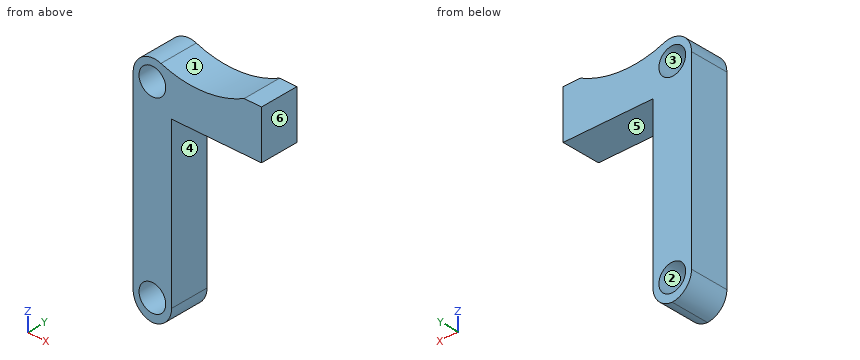
from build123d import *

# Parameters (mm, degrees)
SKETCH1_R           = 3.302
BOSS_EXTRUDE1_DEPTH = 9.525
FILLET1_R           = 5.08
FILLET2_R           = 5.08
FILLET3_DEPTH       = 9.525


with BuildPart() as part:
    # Sketch1 → Boss-Extrude1 (new body)
    with BuildSketch(Plane(origin=(0, 0, 0), x_dir=(1, 0, 0), z_dir=(0, 1, 0))):
        with BuildLine():
            Line((-4.7625, 28.575), (4.7625, 28.575))
            Line((4.7625, 28.575), (4.7625, -17.145))
            Line((4.7625, -17.145), (26.9875, -17.145))
            Line((26.9875, -17.145), (26.9875, -29.1465))
            Line((26.9875, -29.1465), (22.703516651, -29.1465))
            ThreePointArc((22.703516651, -29.1465), (11.1125, -26.347569289), (-0.478516651, -29.1465))
            Line((-0.478516651, -29.1465), (-4.7625, -29.1465))
            Line((-4.7625, -29.1465), (-4.7625, 28.575))
        make_face()
        with Locations(Location((0, -23.241, 0), (0, 0, 90))):
            Circle(SKETCH1_R, mode=Mode.SUBTRACT)
        with Locations(Location((0, 23.241, 0), (0, 0, 90))):
            Circle(SKETCH1_R, mode=Mode.SUBTRACT)
    extrude(amount=BOSS_EXTRUDE1_DEPTH)

    # Fillet1
    # the kernel refuses this fillet: 5.08 mm, written as the material it takes off along each edge
    with BuildSketch(Plane(origin=(-4.7625, -12.7, -28.575), x_dir=(0, 0, 1), z_dir=(0, 1, 0)), Plane(origin=(4.7625, -12.7, -28.575), x_dir=(-1, 0, 0), z_dir=(0, 1, 0))) as fillet1_piece_1:
        with BuildLine():
            CenterArc((FILLET1_R, FILLET1_R), FILLET1_R, 180, 90)
            Line((0, FILLET1_R), (0, 0))
            Line((0, 0), (FILLET1_R, 0))
        make_face()
    extrude(amount=34.925, mode=Mode.SUBTRACT)

    # Fillet2
    # the kernel refuses this fillet: 5.08 mm, written as the material it takes off along each edge
    with BuildSketch(Plane(origin=(-4.7625, -12.543115017, 29.1465), x_dir=(1, 0, 0), z_dir=(0, 1, 0))) as fillet2_piece_1:
        with BuildLine():
            CenterArc((5.08, 5.017246007), FILLET2_R, 180, 80.98481696)
            Line((0, 5.017246007), (-0.1016, 5.017246007))
            Line((-0.1016, 5.017246007), (-0.1016, 0))
            Line((-0.1016, 0), (0, -0.1016))
            ThreePointArc((0, -0.1016), (2.141991675, -0.1016), (4.268063016, -0.10034492))
            Line((4.268063016, -0.10034492), (4.283983349, 0))
        make_face()
    extrude(amount=34.611230034, mode=Mode.SUBTRACT)

    # Fillet3: read off the stored shape, not the designer's step
    # Fillet3 outline → Fillet3 (cut)
    with BuildSketch(Plane(origin=(0, 0, 0), x_dir=(1, 0, 0), z_dir=(0, 1, 0))):
        with BuildLine():
            ThreePointArc((-0.478516651, -29.1465), (0.802955992, -28.533924544), (2.116666667, -27.993938353))
            ThreePointArc((2.116666667, -27.993938353), (-2.569248459, -27.423293904), (-4.7625, -23.243212166))
            Line((-4.7625, -23.243212166), (-4.7625, -24.129253993))
            ThreePointArc((-4.7625, -24.129253993), (-3.545799405, -27.427938232), (-0.478516651, -29.1465))
        make_face()
    extrude(amount=FILLET3_DEPTH, mode=Mode.SUBTRACT)


solid = part.part
Design review of the part built by this model. Coordinates are the model's own, in mm. Face numbers are marked on the shaded views. A direction names the side the tool comes from. Coordinates: 2 decimals unless noted, no trailing zeros. Order: outer loops, then holes, each group sorted by start corner. A loop starts at its lowest first (then second) coordinate and runs counter-clockwise, first axis right, second up.
Item 1: Take a section at C-C, the plane x = 24. Write out the cut boundary in (y, z) (1 decimal).
Item 2: Take a section at D-D, the plane z = 3.5. Write out the cut boundary in (x, y) (1 decimal).
Item 3: For line 1 (Z direction, x = 1, y = 4.75); line 2 (X direction, y = 2, z = -23); line 3 (X direction, y = 4, z = -12.5), list the stretches that pass through material, from the lowest coordinate up.
Item 4: The part is to be moulded in two halves that separate along Z. For the marked faces 1, 2, 3 and 4, say which applies: pulls with the +Z half, pulls with the -Z half, needs draft (parallel to the pull), parting line crosses it, or undercut.
Item 5: Take a section at A-A, the plane y = 3.5. Write out the cut boundary in (x, z) (1 decimal), then the cut area to 3 significant figures.
Item 6: For the marked faces 5 and 6, list the 3-axis set-ups (+Z, -Z, +X, -X, +Y, -Y) from which the entire face can be reached by the end or side of a thin tool; tool diameter is ignored.
Item 7: Take a section at B-B, the plane z = 24. Write out the cut boundary in (x, y) (1 decimal), then the cut area to 3 significant figures.
Item 8: For pin 1 Ø4 at (x, z) = (0, 23.241) entering from -Y; pin 2 Ø5 at (y, z) = (7, 6.5) entering from +X; pin 3 Ø1 at (x, y) = (11.5, 6) entering from -Z (3 decimals); pin 4 Ø2 at (x, z) = (16.5, 23) entering from -Y, all flat-tipped, find the tip position at first contact; note any pin that passes through.
The answers:
1. outline: (0, 17.1) - (9.5, 17.1) - (9.5, 29.1) - (0, 29.1) - close
2. outline: (-4.8, 0) - (4.8, 0) - (4.8, 9.5) - (-4.8, 9.5) - close
3. line 1: z = -28.4 to -26.39, -20.09 to 20.09, 26.39 to 28.28
3. line 2: x = -4.76 to -3.29, 3.29 to 4.76
3. line 3: x = -4.76 to 4.76
4. face 1: pulls with the +Z half
4. face 2: undercut
4. face 3: undercut
4. face 4: needs draft
5. outline: (-4.8, -23.5) arc R5.1 ccw to (0, -28.6) arc R5.1 ccw to (4.8, -23.5) - (4.8, 17.1) - (27, 17.1) - (27, 29.1) - (22.7, 29.1) arc R25.4 cw to (2.1, 28) arc R5.1 ccw to (-4.8, 23.2) - close; hole circle Ø6.6 at (0, -23.2); hole circle Ø6.6 at (0, 23.2)
5. area: 683 mm2
6. face 5: -Z, +X, +Y, -Y
6. face 6: +Z, -Z, +X, +Y, -Y
7. outline: (-4.7, 0) - (-3.2, 0) - (-3.2, 9.5) - (-4.7, 9.5) - close; (3.2, 0) - (27, 0) - (27, 9.5) - (3.2, 9.5) - close
7. area: 241 mm2
8. pin 1: passes through
8. pin 2: stops at x = 4.76
8. pin 3: stops at z = 17.145
8. pin 4: stops at y = 0
